Design review of the part built by this model. Coordinates are the model's own, in mm. Face numbers are marked on the shaded views. A direction names the side the tool comes from. Coordinates: 2 decimals unless noted, no trailing zeros. Write each loop counter-clockwise with the first axis right and the second up, starting at its lowest first coordinate (ties: lowest second). Pieces come first, ordered by that corner, then holes.
Q1. Take a section at B-B, the plane z = 19.5. Write out the cut boundary in (x, y), plus the area to 3 significant figures.
Q2. The part is to be moulded in two halves that separate along Y. For the marked faces 4, 5 and 6, say which applies: released by +Y, released by -Y, zero draft, split by the parting line, or undercut.
Q3. Take a section at A-A, the plane x = 2.2. Write out the cut boundary in (y, z).
Q4. Take a section at D-D, the plane y = -12.5. Write out the cut boundary in (x, z).
Q5. Take a section at C-C, the plane y = -24.5. Write out the cut boundary in (x, z).
Q6. For pin 1 Ø1.6 at (x, y) = (1, -57.5) entering from +Z; pin 2 Ø1 at (x, z) = (1.5, 20) entering from -Y, all flat-tipped, find the tip position at first contact; note any pin that passes through.
Q7. For L1, parallel to Z at x = 1.55, y = -14.5; L2, parallel to Y at x = 1.2, z = 19.5; L3, parallel to Y at x = 1.35, z = 22, list the stretches that pass through material, from the lowest coordinate up.
Q8. For the marked faces 1, 2 and 3, list the 3-axis set-ups (+Z, -Z, +X, -X, +Y, -Y) from which the entire face can be reached by the end or side of a thin tool; tool diameter is ignored.
Autodesk Inventor part; units mm, degrees
ref_plane "YZ Plane" through (0, 0, 0) normal (1, 0, 0) x (0, 1, 0)
ref_plane "XZ Plane" through (0, 0, 0) normal (0, 1, 0) x (-1, 0, 0)
ref_plane "XY Plane" through (0, 0, 0) normal (0, 0, 1) x (1, 0, 0)
sketch "Sketch1" plane through (0, 0, 0) normal (1, 0, 0) x (0, 1, 0)
  line L0 (-92.7646, -8.503) -> (-89.7646, -8.503)
  line L1 (-89.7646, -8.503) -> (-89.7646, -11.753)
  line L2 (-89.7646, -11.753) -> (-92.7646, -11.753)
  line L3 (-92.7646, -11.753) -> (-92.7646, -8.503)
  line L4 (-92.7646, -21.6527) -> (-89.7646, -21.6527)
  line L5 (-89.7646, -21.6527) -> (-89.7646, -21.7527)
  line L6 (-89.7646, -21.7527) -> (-92.7646, -21.7527)
  line L7 (-92.7646, -21.7527) -> (-92.7646, -21.6527)
  line L8 (-56.4516, 8.2437) -> (-59.7016, 8.2437)
  line L9 (-59.7016, 8.2437) -> (-59.7016, 16.2437)
  line L10 (-59.7016, 16.2437) -> (-56.4516, 16.2437)
  line L11 (-56.4516, 16.2437) -> (-56.4516, 8.2437)
  line L12 (-34.4516, 24.2437) -> (-34.4516, 8.2437) construction
  line L13 (-12.4516, 8.2437) -> (-9.2016, 8.2437)
  line L14 (-9.2016, 8.2437) -> (-9.2016, 16.2437)
  line L15 (-9.2016, 16.2437) -> (-12.4516, 16.2437)
  line L16 (-12.4516, 16.2437) -> (-12.4516, 8.2437)
  circle A0 centre (-27.4516, 16.2437) radius 5
  line L17 (-12.4516, 8.2437) -> (-20.4516, 8.2437)
  line L18 (-20.4516, 8.2437) -> (-20.4516, 16.2437)
  line L19 (-20.4516, 16.2437) -> (-12.4516, 16.2437)
  line L20 (-12.4516, 16.2437) -> (-12.4516, 8.2437)
  line L21 (-20.4516, 8.2437) -> (-56.4516, 8.2437)
  line L22 (-56.4516, 8.2437) -> (-56.4516, 24.2437)
  line L23 (-56.4516, 24.2437) -> (-20.4516, 24.2437)
  line L24 (-20.4516, 24.2437) -> (-20.4516, 8.2437)
  point P0 (0, 0)
  dimension "d0" = 3
  dimension "mat" = 3.25
  dimension "d2" = 3
  dimension "kerf" = 0.1
  dimension "d27" = 3.25
  dimension "d28" = 8
  dimension "d29" = 10
  dimension "d34" = 2
  dimension "d35" = 8
  dimension "d38" = 36
extrude "Extrusion5" add sketch "Sketch1" along normal blind 3.25 contours L8 L9 L10 L11 | L11 L22 L23 L24 L18 L21 | L18 L19 L16 L17 | L16 L15 L14 L13
equation "\"d27\" = mat"
equation "\"d36\" = mat"
properties part number "body-side2"
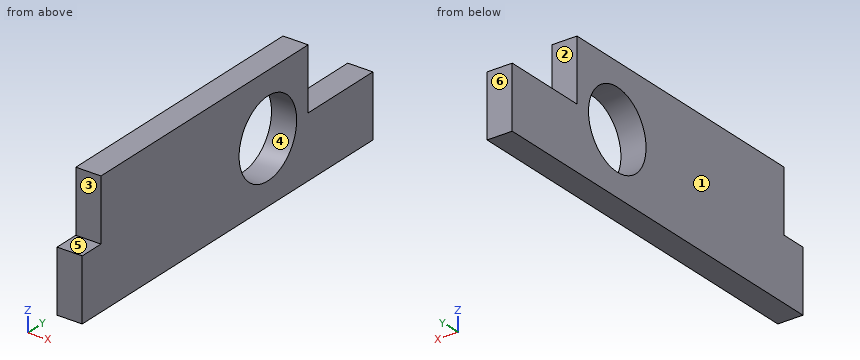
Responses:
1. outline: (0, -56.45) - (3.25, -56.45) - (3.25, -31.25) - (0, -31.25) - close; (0, -23.66) - (3.25, -23.66) - (3.25, -20.45) - (0, -20.45) - close
1. area: 92.3 mm2
2. face 4: undercut
2. face 5: zero draft
2. face 6: released by +Y
3. outline: (-59.7, 8.24) - (-9.2, 8.24) - (-9.2, 16.24) - (-20.45, 16.24) - (-20.45, 24.24) - (-56.45, 24.24) - (-56.45, 16.24) - (-59.7, 16.24) - close; hole circle Ø10 at (-27.45, 16.24)
4. outline: (0, 8.24) - (3.25, 8.24) - (3.25, 16.24) - (0, 16.24) - close
5. outline: (0, 8.24) - (3.25, 8.24) - (3.25, 12.21) - (0, 12.21) - close; (0, 20.28) - (3.25, 20.28) - (3.25, 24.24) - (0, 24.24) - close
6. pin 1: stops at z = 16.24
6. pin 2: stops at y = -56.45
7. L1: z = 8.24 to 16.24
7. L2: y = -56.45 to -31.25, -23.66 to -20.45
7. L3: y = -56.45 to -20.45
8. face 1: +Z, -Z, -X, +Y, -Y
8. face 2: +Z, +X, -X, +Y
8. face 3: +Z, +X, -X, -Y
